Autodesk Inventor part; units mm, degrees
ref_plane "YZ Plane" through (0, 0, 0) normal (1, 0, 0) x (0, 1, 0)
ref_plane "XZ Plane" through (0, 0, 0) normal (0, 1, 0) x (-1, 0, 0)
ref_plane "XY Plane" through (0, 0, 0) normal (0, 0, 1) x (1, 0, 0)
sketch "Skizze2" plane through (0, 0, 0) normal (1, 0, 0) x (0, 1, 0)
  line L0 (0, 0) -> (4.4, 0)
  line L1 (2.5, 6.6) -> (0, 6.6)
  line L2 (0, 6.6) -> (0, 0)
  line L3 (2.5, 6.6) -> (4.4, 0)
  line L4 (-0.88, 0) -> (5.28, 0)
  line L5 (0, 7.92) -> (0, -1.32)
  dimension "d2" = 6.6
  dimension "d3" = 2.5
  dimension "d4" = 4.4
extrude "Extrusion1" add sketch "Skizze2" along normal mid plane 5.8
sketch "Skizze3" plane through (-2.9, 0, 0) normal (0, -1, 0) x (1, 0, 0)
  line L0 (5.8, 0) -> (0, 0)
  line L1 (5.8, 6.6) -> (5.8, 0)
  line L2 (0, 6.6) -> (5.8, 6.6)
  line L3 (0, 0) -> (0, 6.6)
  line L4 (0, 6.6) -> (0, 0) construction
  line L5 (0, 3.3) -> (5.8, 3.3) construction
  line L6 (5.8, 0) -> (5.8, 6.6) construction
  line L7 (0, 6.6) -> (5.8, 6.6) construction
  line L8 (2.9, 6.6) -> (2.9, 0) construction
  circle A0 centre (2.9, 3.3) radius 1.8
  dimension "d7" = 3.6
extrude "Extrusion2" add sketch "Skizze3" along normal blind 4 contours A0
sketch "Skizze4" plane through (2.9, 4.4, 0) normal (0, 0, -1) x (-1, 0, 0)
  line L0 (5.8, 0) -> (0, 0)
  line L1 (0, -4.4) -> (0, 0)
  line L2 (0, -4.4) -> (5.8, -4.4)
  line L3 (5.8, 0) -> (5.8, -4.4)
  line L4 (0, -4.4) -> (0, 0)
  line L5 (0, -3.6) -> (-0.9, -3.6)
  line L6 (-0.9, -3.6) -> (-0.9, -0.2)
  line L7 (-0.9, -0.2) -> (0, -0.2)
  line L8 (0, -0.2) -> (0, -3.6)
  line L9 (5.8, -4.4) -> (0, -4.4)
  line L10 (5.3, -4.4) -> (5.3, -6.4)
  line L11 (5.3, -6.4) -> (0.5, -6.4)
  line L12 (0.5, -6.4) -> (0.5, -4.4)
  line L13 (2.9, -4.4) -> (2.9, 0) construction
  line L14 (5.8, 0) -> (0, 0) construction
  line L15 (4.7, -4.4) -> (4.7, -5.8)
  line L16 (4.7, -5.8) -> (1.1, -5.8)
  line L17 (1.1, -5.8) -> (1.1, -4.4)
  line L18 (0.5, -4.4) -> (1.1, -4.4)
  line L19 (4.7, -4.4) -> (5.3, -4.4)
  line L20 (0, -4.4) -> (5.8, -4.4)
  line L21 (5.8, -1.9) -> (5.8, 0)
  line L22 (5.8, -0.2) -> (6.7, -0.2)
  line L23 (6.7, -0.2) -> (6.7, -3.6)
  line L24 (6.7, -3.6) -> (5.8, -3.6)
  line L25 (5.8, -3.6) -> (5.8, -0.2)
  dimension "d10" = 0.8
  dimension "d11" = 3.4
  dimension "d12" = 0.9
  dimension "d13" = 2
  dimension "d14" = 4.8
  dimension "d16" = 0.6
  dimension "d17" = 0.6
  dimension "d18" = 0.9
extrude "Extrusion3" add sketch "Skizze4" against normal blind 0.2 contours L22 L23 L24 L3 | L1 L5 L6 L7 | L2 L17 L16 L15 L10 L11 L12
fillet "Rundung1" radius 1 1 edges at (0, 2.5, 6.6)
fillet "Rundung2" radius 0.5 1 edges at (-1.8, -4, 3.3)
fillet "Rundung3" radius 0.5 4 edges at (-2.4, -2, 0.1) (2.4, -2, 0.1) (1.8, -1.4, 0.1) (-1.8, -1.4, 0.1)
equation "\"d17\" = d16"
equation "\"d18\" = d12"
properties part number "KT11P4" material "PC/ABS-Kunststoff"
Source: CAD feature listing. Evaluate the final solid. Frame: model axes, mm. A direction names the side the tool comes from. Round coordinates to 2 decimals unless told otherwise and drop trailing zeros. Loops run counter-clockwise (first coordinate to the right, second up) from the corner with the lowest first, then second, coordinate; pieces in that order, holes last. Notation, with made-up numbers: M 83.25,18.25 L 101.25,18.25 A32 ccw 101.25,47.25 Z; hole C 40,85.5 d9. An arc over 180 degrees is marked long. Return JSON: item names as keys, results as strings. Group by question number.
1. Section query A-A on y = -0.5. Output: boundary loops of the cut face in (x, z), and give its area (3 significant figures).
2. Reachability of faces 1 (the face through (3.4, 2.5, 0.2)), 2 (the face through (-0.39, -1.726, 5.057)), 3 (the face through (-3.3, 2.5, 0.2)) from +Z, -Z, +X, -X, +Y, -Y: full face, straight path, thin tool, end or side. Return the list, or none.
3. Section query D-D on x = 2.75. Output: boundary loops of the cut face in (y, z).
4. Section query C-C on z = 3.3. Output: boundary loops of the cut face in (x, y).
5. Section query B-B on x = 0. Output: boundary loops of the cut face in (y, z).
6. Mould query, pull axis Z, two halves, no side actions, for faces 4 (the face through (0, -1.7, 0.2)), 5 (the face through (0, 2, 0)), 6 (the face through (-0.041, 3.542, 2.979)). Classes: released by +Z, released by -Z, zero draft, split by the parting line, or undercut.
7. Pin query (flat end, axial travel): pin 1 (2 mm diameter, centred on x = -3, z = 4.5, fed in from -Y); pin 2 (1 mm diameter, centred on y = 2, z = 5, fed in from -X); pin 3 (3 mm diameter, centred on y = -3, z = 4, fed in from +X). Return the tip coordinate at first contact, or that it passes through.
8. Material intervals for line 1 along X through (y, z) = (1, 3); line 2 along Z through (x, y) = (-3.25, 3.25); line 3 along Y through (x, z) = (-2, 1.5), sorted ascending. Write a range as from..to.
Checks:
{
 "1": {"outline": "M -2.4,0 L -1.8,0 L -1.8,0.2 L -2.4,0.2 Z; C 0,3.3 d3.6; M 1.8,0 L 2.4,0 L 2.4,0.2 L 1.8,0.2 Z", "area": "10.4 mm²"},
 "2": {"face 1": "+Z, +X, +Y, -Y", "face 2": "-Y", "face 3": "+Z, -X, +Y, -Y"},
 "3": {"outline": "M 0,0 L 4.4,0 L 2.71,5.88 A1 ccw 1.75,6.6 L 0,6.6 Z"},
 "4": {"outline": "M -2.9,0 L -1.8,0 L -1.8,-3.5 A0.5 ccw -1.3,-4 L 1.3,-4 A0.5 ccw 1.8,-3.5 L 1.8,0 L 2.9,0 L 2.9,3.45 L -2.9,3.45 Z"},
 "5": {"outline": "M -4,2 A0.5 ccw -3.5,1.5 L 0,1.5 L 0,0 L 4.4,0 L 2.71,5.88 A1 ccw 1.75,6.6 L 0,6.6 L 0,5.1 L -3.5,5.1 A0.5 ccw -4,4.6 Z; M -2,0 L -1.4,0 L -1.4,0.2 L -2,0.2 Z"},
 "6": {"face 4": "undercut", "face 5": "released by -Z", "face 6": "released by +Z"},
 "7": {"pin 1": "stops at y = 0", "pin 2": "stops at x = -2.9", "pin 3": "stops at x = 1.8"},
 "8": {"line 1": "x = -2.9..2.9", "line 2": "z = 0..0.2", "line 3": "y = 0..3.97"}
}
